Here's how the part is built. I have some questions about the finished solid (model axes, mm). A direction names the side the tool comes from. Round coordinates to 2 decimals unless told otherwise and drop trailing zeros. Write each loop counter-clockwise with the first axis right and the second up, starting at its lowest first coordinate (ties: lowest second). Pieces come first, ordered by that corner, then holes. Notation, with made-up numbers: (69, 51) -> (111, 51) arc R28 ccw to (111, 84) -> close; hole circle Ø5 at (26.25, 42.25). An arc over 180 degrees is marked (long way). Answer as CSV lines item,"result".
```python
from build123d import *

# Parameters (mm, degrees)
BOSS_EXTRUDE1_DEPTH = 4
SKETCH2_W           = 10
SKETCH2_H           = 15
CUT_EXTRUDE1_DEPTH  = 4
SKETCH3_R           = 3
CUT_EXTRUDE2_DEPTH  = 2
SKETCH4_R           = 1.5
CUT_EXTRUDE3_DEPTH  = 2


with BuildPart() as part:
    # Sketch1 → Boss-Extrude1 (new body)
    with BuildSketch(Plane(origin=(0, 0, 0), x_dir=(1, 0, 0), z_dir=(0, 1, 0))):
        with BuildLine():
            Line((0, 15), (60, 15))
            ThreePointArc((60, 15), (75, 0), (60, -15))
            Line((60, -15), (0, -15))
            ThreePointArc((0, -15), (-15, 0), (0, 15))
        make_face()
    extrude(amount=BOSS_EXTRUDE1_DEPTH)

    # Sketch2 → Cut-Extrude1 (cut)
    with BuildSketch(Plane(origin=(0, 4, 0), x_dir=(1, 0, 0), z_dir=(0, 1, 0))):
        with Locations((55, 7.5)):
            Rectangle(SKETCH2_W, SKETCH2_H)
    extrude(amount=-CUT_EXTRUDE1_DEPTH, mode=Mode.SUBTRACT)

    # Sketch3 → Cut-Extrude2 (cut)
    with BuildSketch(Plane(origin=(0, 4, 0), x_dir=(1, 0, 0), z_dir=(0, 1, 0))):
        with Locations((-10, 0)):
            Circle(SKETCH3_R)
        with Locations((0, 10)):
            Circle(SKETCH3_R)
        with Locations((10, 0)):
            Circle(SKETCH3_R)
        with Locations((0, -10)):
            Circle(SKETCH3_R)
    extrude(amount=-CUT_EXTRUDE2_DEPTH, mode=Mode.SUBTRACT)

    # Sketch4 → Cut-Extrude3 (cut)
    with BuildSketch(Plane(origin=(0, 2, 0), x_dir=(1, 0, 0), z_dir=(0, 1, 0))):
        with Locations((-10, 0)):
            Circle(SKETCH4_R)
        with Locations((0, 10)):
            Circle(SKETCH4_R)
        with Locations((10, 0)):
            Circle(SKETCH4_R)
        with Locations((0, -10)):
            Circle(SKETCH4_R)
    extrude(amount=-CUT_EXTRUDE3_DEPTH, mode=Mode.SUBTRACT)


solid = part.part
```
1. If I drill on line 1 (Z direction, x = 10, y = 3.05); line 2 (X direction, y = 2.5, z = 0.5); line 3 (X direction, y = 3.25, z = 2), over which ranges is the centre line in solid material (lowest first)?
Numbers:
line 1,"z = -15 to -3, 3 to 15"
line 2,"x = -14.99 to -12.96, -7.04 to 7.04, 12.96 to 74.99"
line 3,"x = -14.87 to -12.24, -7.76 to 7.76, 12.24 to 74.87"
2. On a 3-axis mill with a long thin cutter (end or side, diameter ignored), from which of +Z, -Z, +X, -X, +Y, -Y can I reach the whole of each face in a straight line? I mean faces 1 (the face through (-15, 2, 0)), 2 (the face through (55, 2, 0)), 3 (the face through (-12.4, 3, 1.8)). Say none if no direction works.
Numbers:
face 1,"-X, +Y, -Y"
face 2,"-Z, +Y, -Y"
face 3,"+Y"
3. For pin 1 Ø2.5 at (x, z) = (0, -10) entering from +Y; pin 2 Ø5.5 at (x, z) = (0, 10) entering from +Y; pin 3 Ø1 at (y, z) = (2, 9.5) entering from -X; pin 4 Ø1.2 at (x, y) = (54, 2) entering from -Z, each with a flat end and sliding along its axis, tell me the tip position at first contact or that it passes through.
Numbers:
pin 1,"passes through"
pin 2,"stops at y = 2"
pin 3,"stops at x = -12"
pin 4,"stops at z = 0"
4. Suppose I cut it at B-B on x = 10. Please give me the cut outline in (y, z).
Numbers:
outline,"(0, -15) -> (4, -15) -> (4, -3) -> (2, -3) -> (2, -1.5) -> (0, -1.5) -> close; (0, 1.5) -> (2, 1.5) -> (2, 3) -> (4, 3) -> (4, 15) -> (0, 15) -> close"
5. If we mould it in two halves opening along Z, with no side actions, what happens to faces 4 (the face through (-3, 3, -10)), 5 (the face through (50, 2, -7)), 6 (the face through (25, 2, -15))? For each: released by +Z, released by -Z, zero draft, split by the parting line, or undercut.
Numbers:
face 4,"undercut"
face 5,"zero draft"
face 6,"released by -Z"
6. Suppose I cut it at A-A on y = 1.3. Please give me the cut outline in (x, z), and give its area (3 significant figures).
Numbers:
outline,"(0, -15) -> (50, -15) -> (50, 0) -> (60, 0) -> (60, -15) arc R15 ccw to (60, 15) -> (0, 15) arc R15 ccw to start; hole circle Ø3 at (-10, 0); hole circle Ø3 at (0, -10); hole circle Ø3 at (0, 10); hole circle Ø3 at (10, 0)"
area,"2,330 mm^2"
7. Suppose I cut it at C-C on z = 10. Please give me the cut outline in (x, y).
Numbers:
outline,"(-11.18, 0) -> (-1.5, 0) -> (-1.5, 2) -> (-3, 2) -> (-3, 4) -> (-11.18, 4) -> close; (1.5, 0) -> (71.18, 0) -> (71.18, 4) -> (3, 4) -> (3, 2) -> (1.5, 2) -> close"
8. Suppose I cut it at D-D on x = -5.5. Please give me the cut outline in (y, z), and give its area (3 significant figures).
Numbers:
outline,"(0, -13.96) -> (4, -13.96) -> (4, 13.96) -> (0, 13.96) -> close"
area,"112 mm^2"
